Part model, mm, in its own coordinate system. Face numbers are marked on the shaded views. A direction names the side the tool comes from. Round coordinates to 2 decimals unless told otherwise and drop trailing zeros. Write each loop counter-clockwise with the first axis right and the second up, starting at its lowest first coordinate (ties: lowest second). Pieces come first, ordered by that corner, then holes. Notation, with made-up numbers: M 42.5,72 L 64.5,72 A14 cw 64.5,96 Z; hole C 11.5,35.25 d9. An arc over 180 degrees is marked long. Use one line per item in the form item = value. Start each with the question number.
Item 1: Cut at B-B, the plane y = -125. State how many separate pieces and enclosed holes the cut face has, then the cut area to 3 significant figures.
Item 2: Cut at A-A, the plane x = 0. Give the cut face in (y, z), then the cut area to 3 significant figures.
Item 3: Probe L1, parallel to Y at x = 0, z = 6.75; L2, parallel to X at y = -88, z = 1; L3, parallel to Y at x = 0, z = -3. List the from-to ranges inside material, lowest first.
Item 4: Which spindle directions (+Z, -Z, +X, -X, +Y, -Y) get a long thin tool onto all of the face, cutting with end or side? Do the marked faces 4 and 5. Say none if no direction does.
Item 5: Flat gauge pins, fed straight in: pin 1 Ø5.5 at (y, z) = (-23, 1) entering from -X; pin 2 Ø1 at (x, z) = (0, -2) entering from +Y; pin 3 Ø5 at (x, y) = (130.5, -101.5) entering from -Z. Where does each tip first touch, or does it go through?
Item 6: Cut at C-C, the plane z = -32.5. Give the cut face in (x, y), then the cut area to 3 significant figures.
Item 7: Mould opens along Z. For the marked faces 1, 2 and 3 say: +Z half, -Z half, draft (parallel to the pull), parting line (faces both ways), or undercut.
from build123d import *

# Parameters (mm, degrees)
SKETCH1_R           = 175
BOSS_EXTRUDE4_DEPTH = 15
SKETCH2_R           = 12.5
BOSS_EXTRUDE5_DEPTH = 50
SKETCH3_R           = 25
BOSS_EXTRUDE6_DEPTH = 10


with BuildPart() as part:
    # Sketch1 → Boss-Extrude4 (new, symmetric)
    with BuildSketch(Plane.XY):
        Circle(SKETCH1_R)
        with BuildLine():
            Line((25, -48.733971724), (25, -130.384048104))
            ThreePointArc((25, -130.384048104), (28.914193805, -138.31896858), (37.592592593, -140.042125741))
            ThreePointArc((37.592592593, -140.042125741), (125.573683549, -72.5), (140.076334788, 37.464922691))
            ThreePointArc((140.076334788, 37.464922691), (134.244837518, 44.119057925), (125.415897906, 43.541388957))
            Line((125.415897906, 43.541388957), (54.70485754, 2.716350767))
            ThreePointArc((54.70485754, 2.716350767), (51.30322786, -0.52056309), (49.75404795, -4.953252725))
            ThreePointArc((49.75404795, -4.953252725), (43.301270189, -25), (29.166666667, -40.611643103))
            ThreePointArc((29.166666667, -40.611643103), (26.10243479, -44.169617078), (25, -48.733971724))
        make_face(mode=Mode.SUBTRACT)
        with BuildLine():
            Line((-25, -48.733971724), (-25, -130.384048104))
            ThreePointArc((-25, -130.384048104), (-28.914193805, -138.31896858), (-37.592592593, -140.042125741))
            ThreePointArc((-37.592592593, -140.042125741), (-125.573683549, -72.5), (-140.076334788, 37.464922691))
            ThreePointArc((-140.076334788, 37.464922691), (-134.244837518, 44.119057925), (-125.415897906, 43.541388957))
            Line((-125.415897906, 43.541388957), (-54.70485754, 2.716350767))
            ThreePointArc((-54.70485754, 2.716350767), (-51.30322786, -0.52056309), (-49.75404795, -4.953252725))
            ThreePointArc((-49.75404795, -4.953252725), (-43.301270189, -25), (-29.166666667, -40.611643103))
            ThreePointArc((-29.166666667, -40.611643103), (-26.10243479, -44.169617078), (-25, -48.733971724))
        make_face(mode=Mode.SUBTRACT)
        with BuildLine():
            Line((-29.70485754, 46.017620957), (-100.415897906, 86.842659147))
            ThreePointArc((-100.415897906, 86.842659147), (-105.330643713, 94.199910656), (-102.483742196, 102.57720305))
            ThreePointArc((-102.483742196, 102.57720305), (0, 145), (102.483742196, 102.57720305))
            ThreePointArc((102.483742196, 102.57720305), (105.330643713, 94.199910656), (100.415897906, 86.842659147))
            Line((100.415897906, 86.842659147), (29.70485754, 46.017620957))
            ThreePointArc((29.70485754, 46.017620957), (25.20079307, 44.690180168), (20.587381284, 45.564895829))
            ThreePointArc((20.587381284, 45.564895829), (0, 50), (-20.587381284, 45.564895829))
            ThreePointArc((-20.587381284, 45.564895829), (-25.20079307, 44.690180168), (-29.70485754, 46.017620957))
        make_face(mode=Mode.SUBTRACT)
        with BuildLine():
            Line((-5, -19.364916731), (-5, -24.364916731))
            Line((-5, -24.364916731), (5, -24.364916731))
            Line((5, -24.364916731), (5, -19.364916731))
            ThreePointArc((5, -19.364916731), (0, 20), (-5, -19.364916731))
        make_face(mode=Mode.SUBTRACT)
    extrude(amount=BOSS_EXTRUDE4_DEPTH, both=True)

    # Sketch2 → Boss-Extrude5 (add)
    with BuildSketch(Plane(origin=(0, 0, -15), x_dir=(-1, 0, 0), z_dir=(0, 0, -1))):
        with Locations(Location((0, -125, 0), (0, 0, 180))):
            Circle(SKETCH2_R)
    extrude(amount=BOSS_EXTRUDE5_DEPTH)

    # Sketch3 → Boss-Extrude6 (add)
    with BuildSketch(Plane(origin=(0, 0, -65), x_dir=(-1, 0, 0), z_dir=(0, 0, -1))):
        with Locations((0, -125)):
            Circle(SKETCH3_R)
    extrude(amount=BOSS_EXTRUDE6_DEPTH)

    # Sketch4 → Cut-Revolve1 (revolve, cut)
    with BuildSketch(Plane(origin=(0, 0, 0), x_dir=(1, 0, 0), z_dir=(0, 1, 0)), mode=Mode.PRIVATE) as cut_revolve1_sk:
        Polygon((-175, -10), (-165, 0), (-175, 10), align=None)
    revolve(cut_revolve1_sk.sketch.rotate(Axis((0, 0, 35.70915695), (0, 0, -1)), 180), axis=Axis((0, 0, 35.70915695), (0, 0, -1)), mode=Mode.SUBTRACT)


solid = part.part
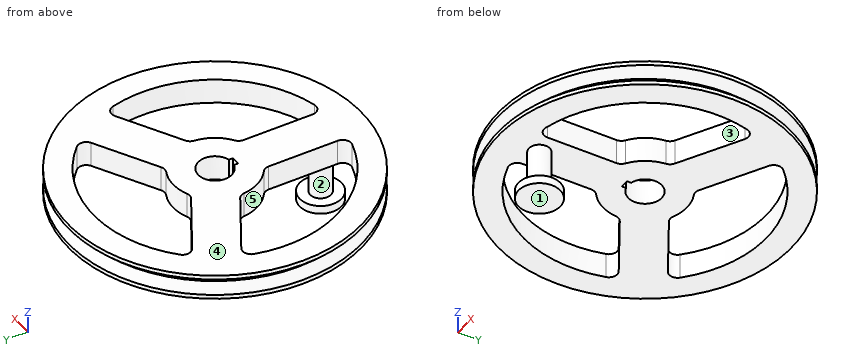
Model answer:
q1.separate_pieces = 3
q1.enclosed_holes = 0
q1.area = 5,900 mm²
q2.outline = M -175,-15 L -137.5,-15 L -137.5,-65 L -150,-65 L -150,-75 L -100,-75 L -100,-65 L -112.5,-65 L -112.5,-15 L -24.36,-15 L -24.36,15 L -175,15 L -175,10 L -165,0 L -175,-10 Z; M 20,-15 L 50,-15 L 50,15 L 20,15 Z; M 145,-15 L 175,-15 L 175,-10 L 165,0 L 175,10 L 175,15 L 145,15 Z
q2.area = 7,870 mm²
q3.L1 = -171.75 to -24.36, 20 to 50, 145 to 171.75
q3.L2 = -140.76 to -115.24, -25 to 25, 115.24 to 140.76
q3.L3 = -168 to -24.36, 20 to 50, 145 to 168
q4.face_4 = +Z, +X, -X, +Y, -Y
q4.face_5 = +Z, -Z
q5.pin_1 = -167.2
q5.pin_2 = 167.5
q5.pin_3 = -15
q6.outline = C 0,-125 d25
q6.area = 491 mm²
q7.face_1 = -Z half
q7.face_2 = undercut
q7.face_3 = draft
